Source: CAD feature listing. Evaluate the final solid. Frame: model axes, mm. Face numbers are marked on the shaded views. A direction names the side the tool comes from. Round coordinates to 2 decimals unless told otherwise and drop trailing zeros. Loops run counter-clockwise (first coordinate to the right, second up) from the corner with the lowest first, then second, coordinate; pieces in that order, holes last. Notation, with made-up numbers: M 50.5,15 L 91.5,15 A29 cw 91.5,49 Z; hole C 51.25,39 d6. An arc over 180 degrees is marked long. Answer as CSV lines item,"result". Start each with the question number.
```python
from build123d import *

# Parameters (mm, degrees)
F0_W     = 126
F0_H     = 78
F1_DEPTH = 2
F2_W     = 126
F2_H     = 78
F2_W_2   = 1.7
F2_H_2   = 75
F3_DEPTH = 19
F5_DEPTH = 100
F6_R     = 0.1


with BuildPart() as f1:
    # F0 (on Top) → F1 (new body)
    with BuildSketch(Plane.XY):
        Rectangle(F0_W, F0_H)
    extrude(amount=F1_DEPTH)

    # F2 (on face) → F3 (join)
    with BuildSketch(Plane.XY.offset(2)):
        Rectangle(F2_W, F2_H)
        Polygon((42.4, 37.5), (61.5, 37.5), (61.5, -37.5), (42.4, -37.5), (40.7, -37.5), (21.6, -37.5), (19.9, -37.5), (0.8, -37.5), (-0.9, -37.5), (-20, -37.5), (-21.7, -37.5), (-40.8, -37.5), (-42.5, -37.5), (-61.5, -37.5), (-61.5, 37.5), (-42.5, 37.5), (-40.8, 37.5), (-21.7, 37.5), (-20, 37.5), (-0.9, 37.5), (0.8, 37.5), (19.9, 37.5), (21.6, 37.5), (40.7, 37.5), align=None, mode=Mode.SUBTRACT)
        with Locations((-41.65, 0)):
            Rectangle(F2_W_2, F2_H_2)
        with Locations((-20.85, 0)):
            Rectangle(F2_W_2, F2_H_2)
        with Locations((-0.05, 0)):
            Rectangle(F2_W_2, F2_H_2)
        with Locations((20.75, 0)):
            Rectangle(F2_W_2, F2_H_2)
        with Locations((41.55, 0)):
            Rectangle(F2_W_2, F2_H_2)
    extrude(amount=F3_DEPTH)

    # F4 (on face) → F5 (cut)
    with BuildSketch(Plane.XZ.offset(39)):
        with BuildLine():
            ThreePointArc((-50.25, 10.5), (-52, 12.25), (-53.75, 10.5))
            Line((-53.75, 10.5), (-50.25, 10.5))
        make_face()
        with BuildLine():
            ThreePointArc((53.75, 10.5), (52, 12.25), (50.25, 10.5))
            Line((50.25, 10.5), (53.75, 10.5))
        make_face()
        with BuildLine():
            Line((53.75, 10.5), (50.25, 10.5))
            ThreePointArc((50.25, 10.5), (52, 8.75), (53.75, 10.5))
        make_face()
        with BuildLine():
            ThreePointArc((33.05, 10.5), (31.3, 12.25), (29.55, 10.5))
            Line((29.55, 10.5), (33.05, 10.5))
        make_face()
        with BuildLine():
            Line((33.05, 10.5), (29.55, 10.5))
            ThreePointArc((29.55, 10.5), (31.3, 8.75), (33.05, 10.5))
        make_face()
        with BuildLine():
            ThreePointArc((12.35, 10.5), (10.6, 12.25), (8.85, 10.5))
            Line((8.85, 10.5), (12.35, 10.5))
        make_face()
        with BuildLine():
            Line((12.35, 10.5), (8.85, 10.5))
            ThreePointArc((8.85, 10.5), (10.6, 8.75), (12.35, 10.5))
        make_face()
        with BuildLine():
            ThreePointArc((-8.85, 10.5), (-10.6, 12.25), (-12.35, 10.5))
            Line((-12.35, 10.5), (-8.85, 10.5))
        make_face()
        with BuildLine():
            Line((-8.85, 10.5), (-12.35, 10.5))
            ThreePointArc((-12.35, 10.5), (-10.6, 8.75), (-8.85, 10.5))
        make_face()
        with BuildLine():
            ThreePointArc((-29.55, 10.5), (-31.3, 12.25), (-33.05, 10.5))
            Line((-33.05, 10.5), (-29.55, 10.5))
        make_face()
        with BuildLine():
            Line((-29.55, 10.5), (-33.05, 10.5))
            ThreePointArc((-33.05, 10.5), (-31.3, 8.75), (-29.55, 10.5))
        make_face()
        with BuildLine():
            Line((-50.25, 10.5), (-53.75, 10.5))
            ThreePointArc((-53.75, 10.5), (-52, 8.75), (-50.25, 10.5))
        make_face()
    extrude(amount=-F5_DEPTH, mode=Mode.SUBTRACT)

    # F6
    f6_edges = [f1.edges().sort_by_distance(p)[0] for p in [
        (-63, -39, 10.5),
        (63, -39, 10.5),
        (63, 39, 10.5),
        (-63, 39, 10.5),
    ]]
    fillet(f6_edges, radius=F6_R)


solid = f1.part
```
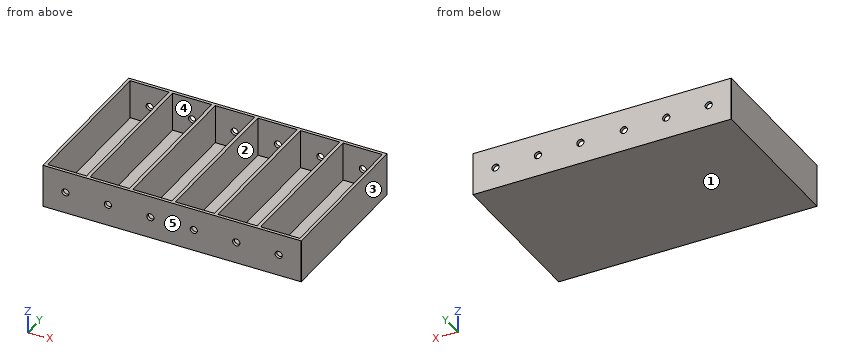
1) Contact query for flat-ended pins moving along their axis: pin 1 Ø5 at (x, y) = (-13, -10) entering from +Z; pin 2 Ø3 at (x, z) = (10.6, 10.5) entering from +Y. Output: stop coordinate, or through.
2) Mould query, pull axis X, two halves, no side actions, for the marked faces 1, 2 and 3. Classes: pulls with the +X half, pulls with the -X half, needs draft (parallel to the pull), parting line crosses it, or undercut.
3) Ray query, line 1 along Y through (x, z) = (56.5, 17); line 2 along Z through (x, y) = (-31, -38); line 3 along Z through (x, y) = (44.5, -21). Return the intervals inside material, ascending.
4) Section B-B, the plane z = 4.5. Give the number of separate pieces and of enclosed holes in the cut face, and give its area (3 significant figures).
5) Section C-C, the plane x = -14.5. Return loops of the section in (y, z), and give its area (3 significant figures).
6) Access query for the marked faces 4 and 5. Directions: +Z, -Z, +X, -X, +Y, -Y. A direction counts if a zero-diameter tool reaches every point of the face in a straight line with its end or side. Return the directions, or none.
7) Section A-A, the plane x = 52. Return loops of the section in (y, z).
8) Section D-D, the plane y = -8. Return loops of the section in (x, z), and give its area (4 significant figures).
Findings below:
1,pin 1,"z = 2"
1,pin 2,"through"
2,face 1,"needs draft"
2,face 2,"undercut"
2,face 3,"pulls with the +X half"
3,line 1,"-39 to -37.5, 37.5 to 39"
3,line 2,"0 to 8.78, 12.22 to 21"
3,line 3,"0 to 2"
4,separate pieces,"1"
4,enclosed holes,"6"
4,area,"1,240 mm²"
5,outline,"M -39,0 L 39,0 L 39,21 L 37.5,21 L 37.5,2 L -37.5,2 L -37.5,21 L -39,21 Z"
5,area,"213 mm²"
6,face 4,"+Z"
6,face 5,"+Z, -Z, +X, -X, -Y"
7,outline,"M -39,0 L 39,0 L 39,8.75 L 37.5,8.75 L 37.5,2 L -37.5,2 L -37.5,8.75 L -39,8.75 Z; M -39,12.25 L -37.5,12.25 L -37.5,21 L -39,21 Z; M 37.5,12.25 L 39,12.25 L 39,21 L 37.5,21 Z"
8,outline,"M -63,0 L 63,0 L 63,21 L 61.5,21 L 61.5,2 L 42.4,2 L 42.4,21 L 40.7,21 L 40.7,2 L 21.6,2 L 21.6,21 L 19.9,21 L 19.9,2 L 0.8,2 L 0.8,21 L -0.9,21 L -0.9,2 L -20,2 L -20,21 L -21.7,21 L -21.7,2 L -40.8,2 L -40.8,21 L -42.5,21 L -42.5,2 L -61.5,2 L -61.5,21 L -63,21 Z"
8,area,"470.5 mm²"
